from build123d import *

# Parameters (mm, degrees)
SKETCH1_R            = 12.1
BOSS_EXTRUDE1_DEPTH  = 3
BOSS_EXTRUDE2_DEPTH  = 3
BOSS_EXTRUDE3_DEPTH  = 3
BOSS_EXTRUDE4_DEPTH  = 3
BOSS_EXTRUDE5_DEPTH  = 3
BOSS_EXTRUDE6_DEPTH  = 3
BOSS_EXTRUDE7_DEPTH  = 3
BOSS_EXTRUDE8_DEPTH  = 3
BOSS_EXTRUDE9_DEPTH  = 3
BOSS_EXTRUDE10_DEPTH = 3
BOSS_EXTRUDE11_DEPTH = 3
BOSS_EXTRUDE12_DEPTH = 3
BOSS_EXTRUDE13_DEPTH = 3
BOSS_EXTRUDE14_DEPTH = 3
BOSS_EXTRUDE15_DEPTH = 3
BOSS_EXTRUDE16_DEPTH = 3
BOSS_EXTRUDE17_DEPTH = 3
BOSS_EXTRUDE18_DEPTH = 3
BOSS_EXTRUDE19_DEPTH = 3
BOSS_EXTRUDE20_DEPTH = 3
BOSS_EXTRUDE21_DEPTH = 3
BOSS_EXTRUDE22_DEPTH = 3
BOSS_EXTRUDE23_DEPTH = 3
BOSS_EXTRUDE24_DEPTH = 3
BOSS_EXTRUDE25_DEPTH = 3


with BuildPart() as part:
    # Sketch1 → Boss-Extrude1 (new body)
    with BuildSketch(Plane.XY):
        Circle(SKETCH1_R)
    extrude(amount=BOSS_EXTRUDE1_DEPTH)

    # Sketch2 → Boss-Extrude2 (add)
    with BuildSketch(Plane.XY):
        Polygon((12.079935981, -0.696524726), (14.645079707, -0.379658233), (14.645079707, 0.379658233), (12.079935981, 0.696524726), align=None)
    extrude(amount=BOSS_EXTRUDE2_DEPTH)

    # Sketch3 → Boss-Extrude3 (add)
    with BuildSketch(Plane.XY):
        Polygon((11.848596009, 2.453726274), (14.244323498, 3.423703853), (14.244323498, 4.157147238), (11.490982299, 3.790425545), align=None)
    extrude(amount=BOSS_EXTRUDE3_DEPTH)

    # Sketch4 → Boss-Extrude4 (add)
    with BuildSketch(Plane.XY):
        Polygon((10.809793799, 5.436759883), (12.872840183, 6.993746179), (12.418878698, 7.595256676), (10.113269073, 6.643176098), align=None)
    extrude(amount=BOSS_EXTRUDE4_DEPTH)

    # Sketch5 → Boss-Extrude5 (add)
    with BuildSketch(Plane.XY):
        Polygon((9.034322006, 8.049287291), (10.624094083, 10.087176261), (9.829208044, 10.707272668), (8.182693208, 8.913671065), align=None)
    extrude(amount=BOSS_EXTRUDE5_DEPTH)

    # Sketch6 → Boss-Extrude6 (add)
    with BuildSketch(Plane.XY):
        Polygon((6.643176098, 10.113269073), (7.651333528, 12.49318195), (7.147254813, 12.706715272), (5.436759883, 10.809793799), align=None)
    extrude(amount=BOSS_EXTRUDE6_DEPTH)

    # Sketch7 → Boss-Extrude7 (add)
    with BuildSketch(Plane.XY):
        Polygon((3.799308717, 11.488048279), (4.157147238, 14.047797936), (3.423703853, 14.047797936), (2.453726274, 11.848596009), align=None)
    extrude(amount=BOSS_EXTRUDE7_DEPTH)

    # Sketch8 → Boss-Extrude8 (add)
    with BuildSketch(Plane.XY):
        Polygon((0.696524726, 12.079935981), (0.379658233, 14.645079707), (-0.379658233, 14.645079707), (-0.696524726, 12.079935981), align=None)
    extrude(amount=BOSS_EXTRUDE8_DEPTH)

    # Sketch9 → Boss-Extrude9 (add)
    with BuildSketch(Plane.XY):
        Polygon((-2.453726274, 11.848596009), (-3.423703853, 14.244323498), (-4.157147238, 14.244323498), (-3.790425545, 11.490982299), align=None)
    extrude(amount=BOSS_EXTRUDE9_DEPTH)

    # Sketch10 → Boss-Extrude10 (add)
    with BuildSketch(Plane.XY):
        Polygon((-5.436759883, 10.809793799), (-6.993746179, 12.872840183), (-7.595256676, 12.418878698), (-6.643176098, 10.113269073), align=None)
    extrude(amount=BOSS_EXTRUDE10_DEPTH)

    # Sketch11 → Boss-Extrude11 (add)
    with BuildSketch(Plane.XY):
        Polygon((-8.049287291, 9.034322006), (-10.087176261, 10.624094083), (-10.707272668, 9.829208044), (-8.913671065, 8.182693208), align=None)
    extrude(amount=BOSS_EXTRUDE11_DEPTH)

    # Sketch12 → Boss-Extrude12 (add)
    with BuildSketch(Plane.XY):
        Polygon((-10.113269073, 6.643176098), (-12.49318195, 7.651333528), (-12.706715272, 7.147254813), (-10.809793799, 5.436759883), align=None)
    extrude(amount=BOSS_EXTRUDE12_DEPTH)

    # Sketch13 → Boss-Extrude13 (add)
    with BuildSketch(Plane.XY):
        Polygon((-11.488048279, 3.799308717), (-14.047797936, 4.157147238), (-14.047797936, 3.423703853), (-11.848596009, 2.453726274), align=None)
    extrude(amount=BOSS_EXTRUDE13_DEPTH)

    # Sketch14 → Boss-Extrude14 (add)
    with BuildSketch(Plane.XY):
        Polygon((-12.079935981, 0.696524726), (-14.645079707, 0.379658233), (-14.645079707, -0.379658233), (-12.079935981, -0.696524726), align=None)
    extrude(amount=BOSS_EXTRUDE14_DEPTH)

    # Sketch15 → Boss-Extrude15 (add)
    with BuildSketch(Plane.XY):
        Polygon((-11.848596009, -2.453726274), (-14.244323498, -3.423703853), (-14.244323498, -4.157147238), (-11.490982299, -3.790425545), align=None)
    extrude(amount=BOSS_EXTRUDE15_DEPTH)

    # Sketch16 → Boss-Extrude16 (add)
    with BuildSketch(Plane.XY):
        Polygon((-10.809793799, -5.436759883), (-12.872840183, -6.993746179), (-12.418878698, -7.595256676), (-10.113269073, -6.643176098), align=None)
    extrude(amount=BOSS_EXTRUDE16_DEPTH)

    # Sketch17 → Boss-Extrude17 (add)
    with BuildSketch(Plane.XY):
        Polygon((-9.034322006, -8.049287291), (-10.624094083, -10.087176261), (-9.829208044, -10.707272668), (-8.182693208, -8.913671065), align=None)
    extrude(amount=BOSS_EXTRUDE17_DEPTH)

    # Sketch18 → Boss-Extrude18 (add)
    with BuildSketch(Plane.XY):
        Polygon((-6.643176098, -10.113269073), (-7.651333528, -12.49318195), (-7.147254813, -12.706715272), (-5.436759883, -10.809793799), align=None)
    extrude(amount=BOSS_EXTRUDE18_DEPTH)

    # Sketch19 → Boss-Extrude19 (add)
    with BuildSketch(Plane.XY):
        Polygon((-3.799308717, -11.488048279), (-4.157147238, -14.047797936), (-3.423703853, -14.047797936), (-2.453726274, -11.848596009), align=None)
    extrude(amount=BOSS_EXTRUDE19_DEPTH)

    # Sketch20 → Boss-Extrude20 (add)
    with BuildSketch(Plane.XY):
        Polygon((-0.696524726, -12.079935981), (-0.696524726, -14.645079707), (0.379658233, -14.645079707), (0.379658233, -12.09404232), align=None)
    extrude(amount=BOSS_EXTRUDE20_DEPTH)

    # Sketch21 → Boss-Extrude21 (add)
    with BuildSketch(Plane.XY):
        Polygon((2.453726274, -11.848596009), (3.423703853, -14.244323498), (4.157147238, -14.244323498), (3.790425545, -11.490982299), align=None)
    extrude(amount=BOSS_EXTRUDE21_DEPTH)

    # Sketch22 → Boss-Extrude22 (add)
    with BuildSketch(Plane.XY):
        Polygon((5.436759883, -10.809793799), (6.993746179, -12.872840183), (7.595256676, -12.418878698), (6.643176098, -10.113269073), align=None)
    extrude(amount=BOSS_EXTRUDE22_DEPTH)

    # Sketch23 → Boss-Extrude23 (add)
    with BuildSketch(Plane.XY):
        Polygon((8.049287291, -9.034322006), (9.863117815, -10.848152529), (10.770033076, -9.941237267), (8.89125817, -8.207041376), align=None)
    extrude(amount=BOSS_EXTRUDE23_DEPTH)

    # Sketch24 → Boss-Extrude24 (add)
    with BuildSketch(Plane.XY):
        Polygon((10.113269073, -6.643176098), (12.49318195, -7.651333528), (12.706715272, -7.147254813), (10.809793799, -5.436759883), align=None)
    extrude(amount=BOSS_EXTRUDE24_DEPTH)

    # Sketch25 → Boss-Extrude25 (add)
    with BuildSketch(Plane.XY):
        Polygon((11.488048279, -3.799308717), (14.047797936, -4.157147238), (14.047797936, -3.423703853), (11.848596009, -2.453726274), align=None)
    extrude(amount=BOSS_EXTRUDE25_DEPTH)


solid = part.part
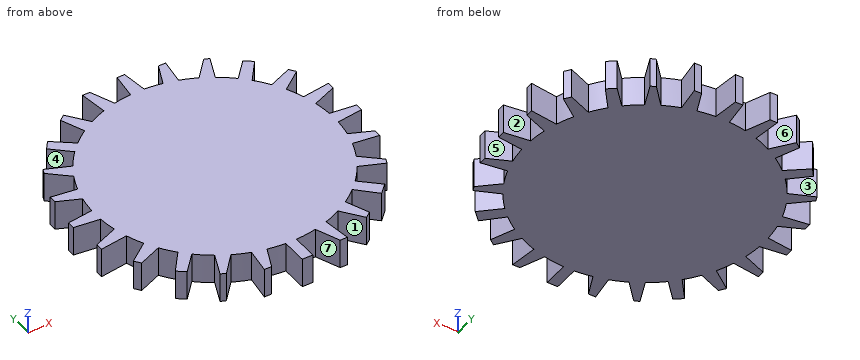
Could you check a few things on this model? Use its own coordinates, in mm. Face numbers are marked on the shaded views. A direction names the side the tool comes from. Give positions to 0.01 mm unless a question says otherwise; leave off trailing zeros. Use CSV: the item, a comma, the result in double quotes. Start each with the question number.
Item 1: For the marked faces 1, 2, 3 and 4, which set-ups out of +Z, -Z, +X, -X, +Y, -Y let a thin tool reach every point of the face, with its end or its side?
Item 2: If I drill on line 1 along X through (y, z) = (-7.5, 1.6); line 2 along X through (y, z) = (-9.5, 0.2); line 3 along Y through (x, z) = (-10.25, 2.2), over which ranges is the centre line in solid material (lowest first)?
Item 3: I'm going to push flat-ended pins straight in: pin 1 (0.8 mm diameter, centred on x = 4, z = 2, fed in from -Y); pin 2 (0.6 mm diameter, centred on y = 4, z = 1, fed in from +X); pin 3 (1 mm diameter, centred on x = 1, z = 2, fed in from -Y). Where does each tip first touch, or does it pass through?
Item 4: If we mould it in two halves opening along Y, with no side actions, what happens to the marked faces 5, 6 and 7? For each: pulls with the +Y half, pulls with the -Y half, needs draft (parallel to the pull), parting line crosses it, or undercut.
Findings:
1,face 1,"+Z, -Z, -Y"
1,face 2,"+Z, -Z, +X"
1,face 3,"+Z, -Z"
1,face 4,"+Z, -Z, -X"
2,line 1,"x = -12.49 to -12.19, -9.5 to 9.5, 12.14 to 12.56"
2,line 2,"x = -10.17 to -8.72, -7.49 to 7.49, 8.51 to 10.29"
2,line 3,"y = -10.38 to -9.61, -6.7 to 6.7, 9.41 to 10.42"
3,pin 1,"stops at y = -14.24"
3,pin 2,"stops at x = 14.24"
3,pin 3,"stops at y = -12.09"
4,face 5,"undercut"
4,face 6,"pulls with the +Y half"
4,face 7,"pulls with the -Y half"
